Verification items for the finished model (mm, model axes). Face numbers are marked on the shaded views. Coordinates: 2 decimals unless noted, no trailing zeros. Write each question's results on one line, items separated by ' | '. Start each with the question number.
(1) Thickness scan on probe 1 along Z at (x, y) = (687, 96); probe 2 along Y at (x, z) = (1412, -13.5); probe 3 along Y at (x, z) = (645, 15). Record the ranges inside material, lowest first. Write a range as [from, to].
(2) Draft check along Y on the marked faces 1 and 2. Enter one of: +Y half, -Y half, draft (parallel to the pull), parting line (faces both ways), or undercut.
(3) Go/stop test with flat-tipped pins: pin 1 (2 mm diameter, centred on x = 1046, y = -18.5, fed in from -Z); pin 2 (5 mm diameter, centred on x = 75.5, y = 134.5, fed in from -Z) (3 decimals); pin 3 (24 mm diameter, centred on x = 81, z = -39, fed in from -Y). Record where each tip stops, or that it passes through.
```python
from build123d import *

# Parameters (mm, degrees)
F1_DEPTH = 285.75


with BuildPart() as f1:
    # F0 (on Right) → F1 (new body)
    with BuildSketch(Plane.YZ):
        with BuildLine():
            Line((139.1939870883, -55.245), (139.1939870883, -0.635))
            ThreePointArc((139.1939870883, -0.635), (139.0079998944, -0.1859871939), (138.5589870883, 0))
            Line((138.5589870883, 0), (-25.2710129117, 0))
            ThreePointArc((-25.2710129117, 0), (-25.7200257177, -0.1859871939), (-25.9060129117, -0.635))
            Line((-25.9060129117, -0.635), (-25.9060129117, -55.245))
            Line((-25.9060129117, -55.245), (-19.4721929117, -55.245))
            Line((-19.4721929117, -55.245), (-19.4721929117, -7.06882))
            ThreePointArc((-19.4721929117, -7.06882), (-19.2862057177, -6.6198071939), (-18.8371929117, -6.43382))
            Line((-18.8371929117, -6.43382), (132.1251670883, -6.43382))
            ThreePointArc((132.1251670883, -6.43382), (132.5741798944, -6.6198071939), (132.7601670883, -7.06882))
            Line((132.7601670883, -7.06882), (132.7601670883, -55.245))
            Line((132.7601670883, -55.245), (139.1939870883, -55.245))
        make_face()
    extrude(amount=F1_DEPTH)

    # F1_face (on face) → F4 section 0
    with BuildSketch(Plane(origin=(285.75, 56.6439870883, -13.4815357622), x_dir=(0, 1, 0), z_dir=(1, 0, 0))):
        with BuildLine():
            ThreePointArc((75.48118, 7.0477157622), (75.9301928061, 6.8617285682), (76.11618, 6.4127157622))
            Line((76.11618, 6.4127157622), (76.11618, -41.7634642378))
            Line((76.11618, -41.7634642378), (82.55, -41.7634642378))
            Line((82.55, -41.7634642378), (82.55, 12.8465357622))
            ThreePointArc((82.55, 12.8465357622), (82.3640128061, 13.2955485682), (81.915, 13.4815357622))
            Line((81.915, 13.4815357622), (-81.915, 13.4815357622))
            ThreePointArc((-81.915, 13.4815357622), (-82.3640128061, 13.2955485682), (-82.55, 12.8465357622))
            Line((-82.55, 12.8465357622), (-82.55, -41.7634642378))
            Line((-82.55, -41.7634642378), (-76.11618, -41.7634642378))
            Line((-76.11618, -41.7634642378), (-76.11618, 6.4127157622))
            ThreePointArc((-76.11618, 6.4127157622), (-75.9301928061, 6.8617285682), (-75.48118, 7.0477157622))
            Line((-75.48118, 7.0477157622), (75.48118, 7.0477157622))
        make_face()
    # F3 (on offset) → F4 section 1
    with BuildSketch(Plane.YZ.offset(692.15)):
        with BuildLine():
            Line((144.325162816, 3.3113971339), (144.325162816, 57.9213971339))
            ThreePointArc((144.325162816, 57.9213971339), (144.1391756221, 58.3704099399), (143.690162816, 58.5563971339))
            Line((143.690162816, 58.5563971339), (-20.139837184, 58.5563971339))
            ThreePointArc((-20.139837184, 58.5563971339), (-20.58884999, 58.3704099399), (-20.774837184, 57.9213971339))
            Line((-20.774837184, 57.9213971339), (-20.774837184, 3.3113971339))
            Line((-20.774837184, 3.3113971339), (-14.341017184, 3.3113971339))
            Line((-14.341017184, 3.3113971339), (-14.341017184, 51.4875771339))
            ThreePointArc((-14.341017184, 51.4875771339), (-14.15502999, 51.9365899399), (-13.706017184, 52.1225771339))
            Line((-13.706017184, 52.1225771339), (137.256342816, 52.1225771339))
            ThreePointArc((137.256342816, 52.1225771339), (137.7053556221, 51.9365899399), (137.891342816, 51.4875771339))
            Line((137.891342816, 51.4875771339), (137.891342816, 3.3113971339))
            Line((137.891342816, 3.3113971339), (144.325162816, 3.3113971339))
        make_face()
    loft()

    # F4_face (on face) → F7 section 0
    with BuildSketch(Plane(origin=(692.15, 61.775162816, 45.0748613717), x_dir=(0, 1, 0), z_dir=(1, 0, 0))):
        with BuildLine():
            ThreePointArc((75.48118, 7.0477157622), (75.9301928061, 6.8617285682), (76.11618, 6.4127157622))
            Line((76.11618, 6.4127157622), (76.11618, -41.7634642378))
            Line((76.11618, -41.7634642378), (82.55, -41.7634642378))
            Line((82.55, -41.7634642378), (82.55, 12.8465357622))
            ThreePointArc((82.55, 12.8465357622), (82.3640128061, 13.2955485682), (81.915, 13.4815357622))
            Line((81.915, 13.4815357622), (-81.915, 13.4815357622))
            ThreePointArc((-81.915, 13.4815357622), (-82.3640128061, 13.2955485682), (-82.55, 12.8465357622))
            Line((-82.55, 12.8465357622), (-82.55, -41.7634642378))
            Line((-82.55, -41.7634642378), (-76.11618, -41.7634642378))
            Line((-76.11618, -41.7634642378), (-76.11618, 6.4127157622))
            ThreePointArc((-76.11618, 6.4127157622), (-75.9301928061, 6.8617285682), (-75.48118, 7.0477157622))
            Line((-75.48118, 7.0477157622), (75.48118, 7.0477157622))
        make_face()
    # F6 (on offset) → F7 section 1
    with BuildSketch(Plane.YZ.offset(1250.95)):
        with BuildLine():
            Line((106.3418790059, -26.1026672399), (106.3418790059, 28.5073327601))
            ThreePointArc((106.3418790059, 28.5073327601), (106.1558918119, 28.9563455661), (105.7068790059, 29.1423327601))
            Line((105.7068790059, 29.1423327601), (-58.1231209941, 29.1423327601))
            ThreePointArc((-58.1231209941, 29.1423327601), (-58.5721338002, 28.9563455661), (-58.7581209941, 28.5073327601))
            Line((-58.7581209941, 28.5073327601), (-58.7581209941, -26.1026672399))
            Line((-58.7581209941, -26.1026672399), (-52.3243009941, -26.1026672399))
            Line((-52.3243009941, -26.1026672399), (-52.3243009941, 22.0735127601))
            ThreePointArc((-52.3243009941, 22.0735127601), (-52.1383138002, 22.5225255661), (-51.6893009941, 22.7085127601))
            Line((-51.6893009941, 22.7085127601), (99.2730590059, 22.7085127601))
            ThreePointArc((99.2730590059, 22.7085127601), (99.7220718119, 22.5225255661), (99.9080590059, 22.0735127601))
            Line((99.9080590059, 22.0735127601), (99.9080590059, -26.1026672399))
            Line((99.9080590059, -26.1026672399), (106.3418790059, -26.1026672399))
        make_face()
    loft()

    # F7_face (on face) → F10 section 0
    with BuildSketch(Plane(origin=(1250.95, 23.7918790059, 15.6607969979), x_dir=(0, 1, 0), z_dir=(1, 0, 0))):
        with BuildLine():
            ThreePointArc((75.48118, 7.0477157622), (75.9301928061, 6.8617285682), (76.11618, 6.4127157622))
            Line((76.11618, 6.4127157622), (76.11618, -41.7634642378))
            Line((76.11618, -41.7634642378), (82.55, -41.7634642378))
            Line((82.55, -41.7634642378), (82.55, 12.8465357622))
            ThreePointArc((82.55, 12.8465357622), (82.3640128061, 13.2955485682), (81.915, 13.4815357622))
            Line((81.915, 13.4815357622), (-81.915, 13.4815357622))
            ThreePointArc((-81.915, 13.4815357622), (-82.3640128061, 13.2955485682), (-82.55, 12.8465357622))
            Line((-82.55, 12.8465357622), (-82.55, -41.7634642378))
            Line((-82.55, -41.7634642378), (-76.11618, -41.7634642378))
            Line((-76.11618, -41.7634642378), (-76.11618, 6.4127157622))
            ThreePointArc((-76.11618, 6.4127157622), (-75.9301928061, 6.8617285682), (-75.48118, 7.0477157622))
            Line((-75.48118, 7.0477157622), (75.48118, 7.0477157622))
        make_face()
    # F9 (on offset) → F10 section 1
    with BuildSketch(Plane.YZ.offset(1555.75)):
        with BuildLine():
            Line((94.718426384, -67.1952603455), (94.718426384, -12.5852603455))
            ThreePointArc((94.718426384, -12.5852603455), (94.5324391901, -12.1362475394), (94.083426384, -11.9502603455))
            Line((94.083426384, -11.9502603455), (-18.946573616, -11.9502603455))
            ThreePointArc((-18.946573616, -11.9502603455), (-19.395586422, -12.1362475394), (-19.581573616, -12.5852603455))
            Line((-19.581573616, -12.5852603455), (-19.581573616, -67.1952603455))
            Line((-19.581573616, -67.1952603455), (-13.147753616, -67.1952603455))
            Line((-13.147753616, -67.1952603455), (-13.147753616, -19.0190803455))
            ThreePointArc((-13.147753616, -19.0190803455), (-12.961766422, -18.5700675394), (-12.512753616, -18.3840803455))
            Line((-12.512753616, -18.3840803455), (87.649606384, -18.3840803455))
            ThreePointArc((87.649606384, -18.3840803455), (88.0986191901, -18.5700675394), (88.284606384, -19.0190803455))
            Line((88.284606384, -19.0190803455), (88.284606384, -67.1952603455))
            Line((88.284606384, -67.1952603455), (94.718426384, -67.1952603455))
        make_face()
    loft()


solid = f1.part
```
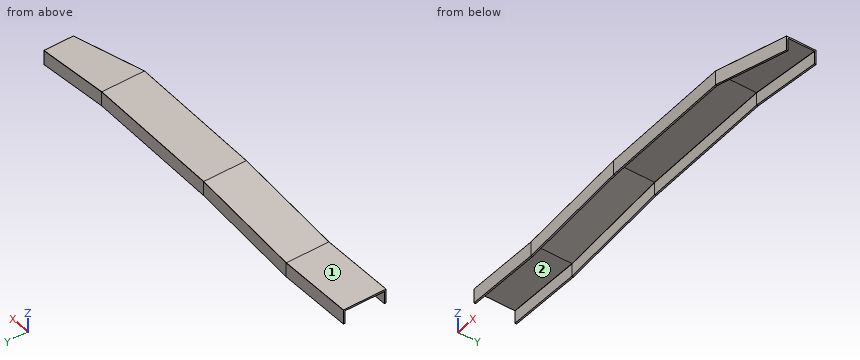
Results are:
1) probe 1: z = [51.38, 57.81] | probe 2: y = [-38.06, -31.62], [93.77, 100.2] | probe 3: y = [-21.37, -14.94], [137.3, 143.73]
2) face 1: draft | face 2: undercut
3) pin 1: stops at z = 33.44 | pin 2: stops at z = -55.245 | pin 3: stops at y = -25.91
